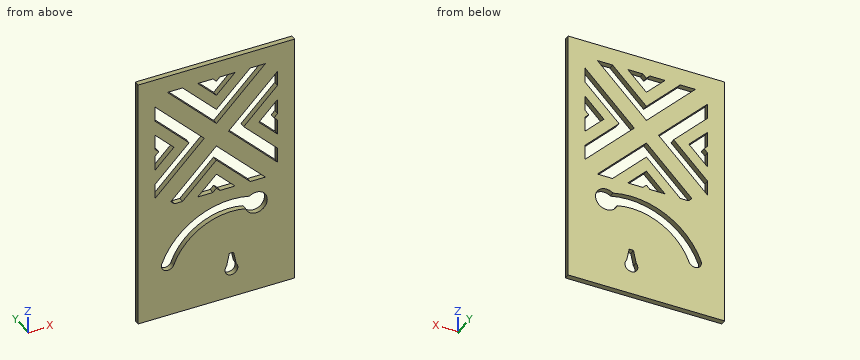
```python
from build123d import *

# Parameters (mm, degrees)
IZIM1_W                     = 73
IZIM1_H                     = 120
Y_KSEKLIK_EKSTR_ZYON1_DEPTH = 2.5
KES_EKSTR_ZYON2_DEPTH       = 3.5
IZIM5_R                     = 3
KES_EKSTR_ZYON3_DEPTH       = 3.5
IZIM6_R                     = 5.15
KES_EKSTR_ZYON4_DEPTH       = 3.5
KES_EKSTR_ZYON5_DEPTH       = 3.5


with BuildPart() as part:
    # Çizim1 → Yükseklik-Ekstrüzyon1 (new body)
    with BuildSketch(Plane(origin=(0, 0, 0), x_dir=(1, 0, 0), z_dir=(0, 1, 0))):
        with Locations((36.5, 60)):
            Rectangle(IZIM1_W, IZIM1_H)
    extrude(amount=Y_KSEKLIK_EKSTR_ZYON1_DEPTH)

    # Çizim4 → Kes-Ekstrüzyon2 (cut, through all)
    with BuildSketch(Plane.XZ):
        with BuildLine():
            Line((41.258359694, -104.027018589), (42.500062903, -98.009051571))
            Line((42.500062903, -98.009051571), (44.499937097, -98.031483944))
            Line((44.499937097, -98.031483944), (45.758359694, -104.045976978))
            ThreePointArc((45.758359694, -104.045976978), (43.487361186, -109.020744393), (41.258359694, -104.027018589))
        make_face()
    extrude(amount=-KES_EKSTR_ZYON2_DEPTH, mode=Mode.SUBTRACT)

    # Çizim5 → Kes-Ekstrüzyon3 (cut, through all)
    with BuildSketch(Plane.XZ):
        with Locations((13.856266363, -94.455359404)):
            Circle(IZIM5_R)
        with BuildLine():
            ThreePointArc((53.975019366, -79.171862015), (52.270586975, -75.286645133), (56.155803858, -73.582212742))
            ThreePointArc((56.155803858, -73.582212742), (29.511480202, -74.134241759), (11.061441726, -93.364967158))
            ThreePointArc((11.061441726, -93.364967158), (14.411030317, -91.507099417), (16.856266363, -94.455359404))
            ThreePointArc((16.856266363, -94.455359404), (16.804526351, -95.010123359), (16.651091, -95.54575165))
            ThreePointArc((16.651091, -95.54575165), (31.921911605, -79.628768168), (53.975019366, -79.171862015))
        make_face()
        with Locations((55.065411612, -76.377037379)):
            Circle(IZIM5_R)
    extrude(amount=-KES_EKSTR_ZYON3_DEPTH, mode=Mode.SUBTRACT)

    # Çizim6 → Kes-Ekstrüzyon4 (cut, through all)
    with BuildSketch(Plane.XZ):
        with Locations((55.065411612, -76.377037379)):
            Circle(IZIM6_R)
    extrude(amount=-KES_EKSTR_ZYON4_DEPTH, mode=Mode.SUBTRACT)

    # Çizim7 → Kes-Ekstrüzyon5 (cut, through all)
    with BuildSketch(Plane.XZ):
        Polygon((16.916738879, -65), (20.727922061, -65), (22.357864376, -63.370057685), (18.82233047, -59.834523779), (15.286796564, -63.370057685), align=None)
        Polygon((22.357864376, -63.370057685), (25.893398282, -59.834523779), (22.357864376, -56.298989873), (18.82233047, -59.834523779), align=None)
        Polygon((25.893398282, -59.834523779), (29.428932188, -56.298989873), (25.893398282, -52.763455967), (22.357864376, -56.298989873), align=None)
        Polygon((29.428932188, -56.298989873), (32.964466094, -52.763455967), (29.428932188, -49.227922061), (25.893398282, -52.763455967), align=None)
        Polygon((32.964466094, -52.763455967), (36.5, -49.227922061), (32.964466094, -45.692388155), (29.428932188, -49.227922061), align=None)
        Polygon((36.5, -49.227922061), (40.035533906, -45.692388155), (36.5, -42.156854249), (32.964466094, -45.692388155), align=None)
        Polygon((40.035533906, -52.763455967), (43.571067812, -49.227922061), (40.035533906, -45.692388155), (36.5, -49.227922061), align=None)
        Polygon((43.571067812, -56.298989873), (47.106601718, -52.763455967), (43.571067812, -49.227922061), (40.035533906, -52.763455967), align=None)
        Polygon((47.106601718, -59.834523779), (50.642135624, -56.298989873), (47.106601718, -52.763455967), (43.571067812, -56.298989873), align=None)
        Polygon((50.642135624, -63.370057685), (54.17766953, -59.834523779), (50.642135624, -56.298989873), (47.106601718, -59.834523779), align=None)
        Polygon((52.272077939, -65), (56.083261121, -65), (57.713203436, -63.370057685), (54.17766953, -59.834523779), (50.642135624, -63.370057685), align=None)
        Polygon((56.083261121, -65), (59.343145751, -65), (57.713203436, -63.370057685), align=None)
        Polygon((41.941125497, -65), (45.201010127, -65), (43.571067812, -63.370057685), align=None)
        Polygon((38.129942315, -65), (41.941125497, -65), (43.571067812, -63.370057685), (40.035533906, -59.834523779), (36.5, -63.370057685), align=None)
        Polygon((36.5, -63.370057685), (40.035533906, -59.834523779), (36.5, -56.298989873), (32.964466094, -59.834523779), align=None)
        Polygon((31.058874503, -65), (34.870057685, -65), (36.5, -63.370057685), (32.964466094, -59.834523779), (29.428932188, -63.370057685), align=None)
        Polygon((27.798989873, -65), (31.058874503, -65), (29.428932188, -63.370057685), align=None)
        Polygon((8, -52.272077939), (8, -59.343145751), (13.165476221, -54.17766953), (9.629942315, -50.642135624), align=None)
        Polygon((9.629942315, -50.642135624), (13.165476221, -54.17766953), (16.701010127, -50.642135624), (13.165476221, -47.106601718), align=None)
        Polygon((13.165476221, -47.106601718), (16.701010127, -50.642135624), (20.236544033, -47.106601718), (16.701010127, -43.571067812), align=None)
        Polygon((16.701010127, -43.571067812), (20.236544033, -47.106601718), (23.772077939, -43.571067812), (20.236544033, -40.035533906), align=None)
        Polygon((20.236544033, -40.035533906), (23.772077939, -43.571067812), (27.307611845, -40.035533906), (23.772077939, -36.5), align=None)
        Polygon((23.772077939, -36.5), (27.307611845, -40.035533906), (30.843145751, -36.5), (27.307611845, -32.964466094), align=None)
        Polygon((20.236544033, -32.964466094), (23.772077939, -36.5), (27.307611845, -32.964466094), (23.772077939, -29.428932188), align=None)
        Polygon((16.701010127, -29.428932188), (20.236544033, -32.964466094), (23.772077939, -29.428932188), (20.236544033, -25.893398282), align=None)
        Polygon((13.165476221, -25.893398282), (16.701010127, -29.428932188), (20.236544033, -25.893398282), (16.701010127, -22.357864376), align=None)
        Polygon((9.629942315, -22.357864376), (13.165476221, -25.893398282), (16.701010127, -22.357864376), (13.165476221, -18.82233047), align=None)
        Polygon((8, -16.916738879), (8, -20.727922061), (9.629942315, -22.357864376), (13.165476221, -18.82233047), (9.629942315, -15.286796564), align=None)
        Polygon((8, -13.656854249), (8, -16.916738879), (9.629942315, -15.286796564), align=None)
        Polygon((8, -41.941125497), (8, -45.201010127), (9.629942315, -43.571067812), align=None)
        Polygon((8, -38.129942315), (8, -41.941125497), (9.629942315, -43.571067812), (13.165476221, -40.035533906), (9.629942315, -36.5), align=None)
        Polygon((9.629942315, -36.5), (13.165476221, -40.035533906), (16.701010127, -36.5), (13.165476221, -32.964466094), align=None)
        Polygon((8, -31.058874503), (8, -34.870057685), (9.629942315, -36.5), (13.165476221, -32.964466094), (9.629942315, -29.428932188), align=None)
        Polygon((8, -27.798989873), (8, -31.058874503), (9.629942315, -29.428932188), align=None)
        Polygon((63.370057685, -57.713203436), (65, -59.343145751), (65, -56.083261121), align=None)
        Polygon((63.370057685, -57.713203436), (65, -56.083261121), (65, -52.272077939), (63.370057685, -50.642135624), (59.834523779, -54.17766953), align=None)
        Polygon((56.298989873, -50.642135624), (59.834523779, -54.17766953), (63.370057685, -50.642135624), (59.834523779, -47.106601718), align=None)
        Polygon((52.763455967, -47.106601718), (56.298989873, -50.642135624), (59.834523779, -47.106601718), (56.298989873, -43.571067812), align=None)
        Polygon((49.227922061, -43.571067812), (52.763455967, -47.106601718), (56.298989873, -43.571067812), (52.763455967, -40.035533906), align=None)
        Polygon((45.692388155, -40.035533906), (49.227922061, -43.571067812), (52.763455967, -40.035533906), (49.227922061, -36.5), align=None)
        Polygon((42.156854249, -36.5), (45.692388155, -40.035533906), (49.227922061, -36.5), (45.692388155, -32.964466094), align=None)
        Polygon((45.692388155, -32.964466094), (49.227922061, -36.5), (52.763455967, -32.964466094), (49.227922061, -29.428932188), align=None)
        Polygon((49.227922061, -29.428932188), (52.763455967, -32.964466094), (56.298989873, -29.428932188), (52.763455967, -25.893398282), align=None)
        Polygon((52.763455967, -25.893398282), (56.298989873, -29.428932188), (59.834523779, -25.893398282), (56.298989873, -22.357864376), align=None)
        Polygon((56.298989873, -22.357864376), (59.834523779, -25.893398282), (63.370057685, -22.357864376), (59.834523779, -18.82233047), align=None)
        Polygon((63.370057685, -22.357864376), (65, -20.727922061), (65, -13.656854249), (59.834523779, -18.82233047), align=None)
        Polygon((56.298989873, -36.5), (59.834523779, -40.035533906), (63.370057685, -36.5), (59.834523779, -32.964466094), align=None)
        Polygon((63.370057685, -43.571067812), (65, -41.941125497), (65, -38.129942315), (63.370057685, -36.5), (59.834523779, -40.035533906), align=None)
        Polygon((63.370057685, -36.5), (65, -34.870057685), (65, -31.058874503), (63.370057685, -29.428932188), (59.834523779, -32.964466094), align=None)
        Polygon((63.370057685, -29.428932188), (65, -31.058874503), (65, -27.798989873), align=None)
        Polygon((63.370057685, -43.571067812), (65, -45.201010127), (65, -41.941125497), align=None)
        Polygon((22.357864376, -9.629942315), (20.727922061, -8), (13.656854249, -8), (18.82233047, -13.165476221), align=None)
        Polygon((22.357864376, -16.701010127), (25.893398282, -13.165476221), (22.357864376, -9.629942315), (18.82233047, -13.165476221), align=None)
        Polygon((25.893398282, -20.236544033), (29.428932188, -16.701010127), (25.893398282, -13.165476221), (22.357864376, -16.701010127), align=None)
        Polygon((29.428932188, -23.772077939), (32.964466094, -20.236544033), (29.428932188, -16.701010127), (25.893398282, -20.236544033), align=None)
        Polygon((32.964466094, -27.307611845), (36.5, -23.772077939), (32.964466094, -20.236544033), (29.428932188, -23.772077939), align=None)
        Polygon((40.035533906, -27.307611845), (43.571067812, -23.772077939), (40.035533906, -20.236544033), (36.5, -23.772077939), align=None)
        Polygon((43.571067812, -23.772077939), (47.106601718, -20.236544033), (43.571067812, -16.701010127), (40.035533906, -20.236544033), align=None)
        Polygon((47.106601718, -20.236544033), (50.642135624, -16.701010127), (47.106601718, -13.165476221), (43.571067812, -16.701010127), align=None)
        Polygon((50.642135624, -16.701010127), (54.17766953, -13.165476221), (50.642135624, -9.629942315), (47.106601718, -13.165476221), align=None)
        Polygon((57.713203436, -9.629942315), (56.083261121, -8), (52.272077939, -8), (50.642135624, -9.629942315), (54.17766953, -13.165476221), align=None)
        Polygon((43.571067812, -9.629942315), (41.941125497, -8), (38.129942315, -8), (36.5, -9.629942315), (40.035533906, -13.165476221), align=None)
        Polygon((36.5, -16.701010127), (40.035533906, -13.165476221), (36.5, -9.629942315), (32.964466094, -13.165476221), align=None)
        Polygon((36.5, -9.629942315), (34.870057685, -8), (31.058874503, -8), (29.428932188, -9.629942315), (32.964466094, -13.165476221), align=None)
        Polygon((57.713203436, -9.629942315), (59.343145751, -8), (56.083261121, -8), align=None)
        Polygon((29.428932188, -9.629942315), (31.058874503, -8), (27.798989873, -8), align=None)
        Polygon((36.5, -30.843145751), (40.035533906, -27.307611845), (36.5, -23.772077939), (32.964466094, -27.307611845), align=None)
        Polygon((43.571067812, -9.629942315), (45.201010127, -8), (41.941125497, -8), align=None)
    extrude(amount=-KES_EKSTR_ZYON5_DEPTH, mode=Mode.SUBTRACT)


solid = part.part
```
Source: CAD feature listing. Evaluate the final solid. Frame: model axes, mm. Coordinates: 2 decimals unless noted, no trailing zeros. Loops run counter-clockwise (first coordinate to the right, second up) from the corner with the lowest first, then second, coordinate; pieces in that order, holes last. Notation, with made-up numbers: (16, 33) -> (67, 33) arc R33 ccw to (67, 68) -> close; hole circle Ø3 at (-1, -27.5). An arc over 180 degrees is marked (long way). One line per item, written item: value. Start each with the question number.
Q1. Section query A-A, the plane z = -53.5. Return the cut outline in (x, y), and give its area (3 significant figures).
Q2. Section query C-C, the plane y = 0.75. Give the number of separate pieces and of enclosed holes in the cut face, and give its area (3 significant figures).
Q3. Section query B-B, the plane z = -74.5. Return the cut outline in (x, y).
Q4. Line query: line 1 along Z through (x, y) = (31, 1.05); line 2 along Z through (x, y) = (10.5, 0.9); line 3 along Z through (x, y) = (47.5, 0.4). Output: solid intervals per line, ascending.
Q5. Section query D-D, the plane z = -102.5. Return the cut outline in (x, y), and give its area (3 significant figures).
Results:
1. outline: (0, 0) -> (8, 0) -> (8, 2.5) -> (0, 2.5) -> close; (13.84, 0) -> (25.16, 0) -> (25.16, 2.5) -> (13.84, 2.5) -> close; (32.23, 0) -> (40.77, 0) -> (40.77, 2.5) -> (32.23, 2.5) -> close; (47.84, 0) -> (59.16, 0) -> (59.16, 2.5) -> (47.84, 2.5) -> close; (65, 0) -> (73, 0) -> (73, 2.5) -> (65, 2.5) -> close
1. area: 118 mm^2
2. separate pieces: 1
2. enclosed holes: 10
2. area: 6,970 mm^2
3. outline: (0, 0) -> (28.71, 0) -> (28.71, 2.5) -> (0, 2.5) -> close; (59.86, 0) -> (73, 0) -> (73, 2.5) -> (59.86, 2.5) -> close
4. line 1: -120 to -80.05, -73.52 to -65, -61.8 to -54.73, -47.66 to -25.34, -18.27 to -11.2, -8 to 0
4. line 2: -120 to -56.84, -49.77 to -42.7, -30.3 to -23.23, -16.16 to 0
4. line 3: -120 to -77.48, -71.43 to -60.23, -53.16 to -41.84, -31.16 to -19.84, -12.77 to 0
5. outline: (0, 0) -> (41.57, 0) -> (41.57, 2.5) -> (0, 2.5) -> close; (45.43, 0) -> (73, 0) -> (73, 2.5) -> (45.43, 2.5) -> close
5. area: 173 mm^2
